Source: CAD feature listing. Evaluate the final solid. Frame: model axes, mm. Coordinates: 2 decimals unless noted, no trailing zeros. Loops run counter-clockwise (first coordinate to the right, second up) from the corner with the lowest first, then second, coordinate; pieces in that order, holes last. Notation, with made-up numbers: (23.5, 85.5) - (40.5, 85.5) arc R21 ccw to (40.5, 115.5) - close; hole circle Ø8 at (-17.5, 37). An arc over 180 degrees is marked (long way). Use CSV: the item, a comma, the result in double quotes. Start each with the question number.
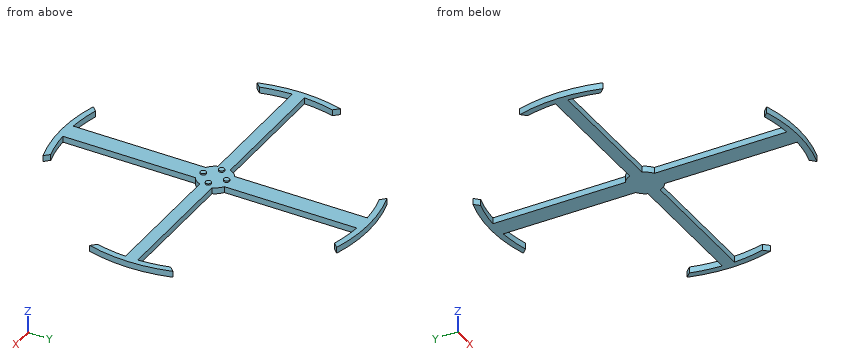
```python
from build123d import *

# Parameters (mm, degrees)
F1_DEPTH = 5
F3_DEPTH = 5
F4_R     = 2.25
F5_DEPTH = 1.2


with BuildPart() as f1:
    # F0 (on Top) → F1 (new body)
    with BuildSketch(Plane.XY):
        with BuildLine():
            ThreePointArc((-116.2578831103, -29.7338967292), (-118.7227043002, -17.4619438679), (-119.8957880828, -5))
            Line((-119.8957880828, -5), (-7.5, -5))
            Line((-7.5, -5), (-7.5, -119.76539567))
            ThreePointArc((-7.5, -119.76539567), (-19.9347609629, -118.3326045744), (-32.152625953, -115.6123204694))
            Line((-32.152625953, -115.6123204694), (-36.1232570919, -119.6666632654))
            ThreePointArc((-36.1232570919, -119.6666632654), (0, -125), (36.1232570919, -119.6666632654))
            Line((36.1232570919, -119.6666632654), (32.152625953, -115.6123204694))
            ThreePointArc((32.152625953, -115.6123204694), (19.9347609629, -118.3326045744), (7.5, -119.76539567))
            Line((7.5, -119.76539567), (7.5, -5))
            Line((7.5, -5), (119.8957880828, -5))
            ThreePointArc((119.8957880828, -5), (118.7227043002, -17.4619438679), (116.2578831103, -29.7338967292))
            Line((116.2578831103, -29.7338967292), (120.3204231937, -33.8820861591))
            ThreePointArc((120.3204231937, -33.8820861591), (125, 0), (120.3204231937, 33.8820861591))
            Line((120.3204231937, 33.8820861591), (116.2578831103, 29.7338967292))
            ThreePointArc((116.2578831103, 29.7338967292), (118.7227043002, 17.4619438679), (119.8957880828, 5))
            Line((119.8957880828, 5), (7.5, 5))
            Line((7.5, 5), (7.5, 119.76539567))
            ThreePointArc((7.5, 119.76539567), (19.9347609629, 118.3326045744), (32.152625953, 115.6123204694))
            Line((32.152625953, 115.6123204694), (36.1232570919, 119.6666632654))
            ThreePointArc((36.1232570919, 119.6666632654), (0, 125), (-36.1232570919, 119.6666632654))
            Line((-36.1232570919, 119.6666632654), (-32.152625953, 115.6123204694))
            ThreePointArc((-32.152625953, 115.6123204694), (-19.9347609629, 118.3326045744), (-7.5, 119.76539567))
            Line((-7.5, 119.76539567), (-7.5, 5))
            Line((-7.5, 5), (-119.8957880828, 5))
            ThreePointArc((-119.8957880828, 5), (-118.7227043002, 17.4619438679), (-116.2578831103, 29.7338967292))
            Line((-116.2578831103, 29.7338967292), (-120.3204231937, 33.8820861591))
            ThreePointArc((-120.3204231937, 33.8820861591), (-125, 0), (-120.3204231937, -33.8820861591))
            Line((-120.3204231937, -33.8820861591), (-116.2578831103, -29.7338967292))
        make_face()
    extrude(amount=F1_DEPTH)

    # F2 (on face) → F3 (join)
    with BuildSketch(Plane(origin=(0, 0, 0), x_dir=(1, 0, 0), z_dir=(0, 0, -1))):
        with BuildLine():
            Line((7.5, 5), (13.0766968306, 5))
            ThreePointArc((13.0766968306, 5), (10.8389869024, 8.8609459387), (7.5, 11.8215904175))
            Line((7.5, 11.8215904175), (7.5, 5))
        make_face()
        with BuildLine():
            ThreePointArc((7.5, -11.8215904175), (10.8389869024, -8.8609459387), (13.0766968306, -5))
            Line((13.0766968306, -5), (7.5, -5))
            Line((7.5, -5), (7.5, -11.8215904175))
        make_face()
        with BuildLine():
            ThreePointArc((-13.0766968306, -5), (-10.8389869024, -8.8609459387), (-7.5, -11.8215904175))
            Line((-7.5, -11.8215904175), (-7.5, -5))
            Line((-7.5, -5), (-13.0766968306, -5))
        make_face()
        with BuildLine():
            Line((-7.5, 5), (-7.5, 11.8215904175))
            ThreePointArc((-7.5, 11.8215904175), (-10.8389869024, 8.8609459387), (-13.0766968306, 5))
            Line((-13.0766968306, 5), (-7.5, 5))
        make_face()
    extrude(amount=-F3_DEPTH)

    # F4 (on face) → F5 (join)
    with BuildSketch(Plane.XY.offset(5)):
        with Locations((0, 9.5)):
            Circle(F4_R)
        with Locations((-9.5, 0)):
            Circle(F4_R)
        with Locations((0, -9.5)):
            Circle(F4_R)
        with Locations((9.5, 0)):
            Circle(F4_R)
    extrude(amount=F5_DEPTH)


solid = f1.part
```
(1) Ray query, line 1 (X direction, y = 12, z = 0.5); line 2 (X direction, y = 11, z = 4.5); line 3 (Y direction, x = 19, z = 2.25). Return the intervals inside material, ascending. Write a range as [from, to].
(2) Pin query (flat end, axial travel): pin 1 Ø1.5 at (y, z) = (-19.5, 0.5) entering from +X; pin 2 Ø1.5 at (y, z) = (-73.5, 3.5) entering from +X; pin 3 Ø1.5 at (y, z) = (62, 3) entering from -X. Return the tip coordinate at first contact, or that it passes through.
(3) Section A-A on y = 15. Output: boundary loops of the cut face in (x, z).
(4) Section D-D on y = 97.5. Output: boundary loops of the cut face in (x, z).
(5) Section C-C on x = -25. Output: boundary loops of the cut face in (y, z), plus the area to 3 significant figures.
Solution:
1,line 1,"x = [-124.42, -119.4], [-7.5, 7.5], [119.4, 124.42]"
1,line 2,"x = [-124.52, -119.49], [-8.66, 8.66], [119.49, 124.52]"
1,line 3,"y = [-123.55, -118.49], [-5, 5], [118.49, 123.55]"
2,pin 1,"stops at x = 123.59"
2,pin 2,"stops at x = 7.5"
2,pin 3,"stops at x = -7.5"
3,outline,"(-124.1, 0) - (-119.06, 0) - (-119.06, 5) - (-124.1, 5) - close; (-7.5, 0) - (7.5, 0) - (7.5, 5) - (-7.5, 5) - close; (119.06, 0) - (124.1, 0) - (124.1, 5) - (119.06, 5) - close"
4,outline,"(-7.5, 0) - (7.5, 0) - (7.5, 5) - (-7.5, 5) - close"
5,outline,"(-122.47, 0) - (-117.37, 0) - (-117.37, 5) - (-122.47, 5) - close; (-5, 0) - (5, 0) - (5, 5) - (-5, 5) - close; (117.37, 0) - (122.47, 0) - (122.47, 5) - (117.37, 5) - close"
5,area,"101 mm²"
